Could you check a few things on this model? Use its own coordinates, in mm. Coordinates: 2 decimals unless noted, no trailing zeros. Order: outer loops, then holes, each group sorted by start corner. A loop starts at its lowest first (then second) coordinate and runs counter-clockwise, first axis right, second up. Notation, with made-up numbers: M -36.75,-28.5 L 6.25,-28.5 A19 ccw 6.25,-24.5 Z; hole C 26,-31 d8. An arc over 180 degrees is marked long. Put each result on its own line as item: value. Start each with the question number.
Solid Edge part; units mm, degrees
sketch "Sketch1" plane through (0, 0, 0) normal (0, 0, 1) x (1, 0, 0)
  line L0 (-0.1, 7.1216) -> (-0.1, 2.6716)
  line L1 (7.2, 2.6716) -> (-0.1, 2.6716)
  line L2 (7.2, 2.6716) -> (7.2, 0.455)
  line L3 (-0.1, 0.455) -> (7.2, 0.455)
  line L4 (-0.1, 0.455) -> (-0.1, 0)
  line L5 (9.2723, 0) -> (-0.1, 0)
  line L6 (6.623, 7.1216) -> (9.2723, 0)
  line L7 (6.623, 7.1216) -> (-0.1, 7.1216)
  dimension "D1" = 0.1
  dimension "D2" = 0.1
  dimension "D3" = 7.2
extrude "Protrusion1" add sketch "Sketch1" along normal blind 0.1
sketch "Sketch2" plane through (4.6037, 3.5608, 0.1) normal (0, 0, 1) x (1, 0, 0)
  line L0 (-2.7487, 0.3108) -> (-2.0887, 0.3108)
  line L1 (-2.0887, 0.3108) -> (-2.0887, 1.7108)
  line L2 (-2.0887, 1.7108) -> (-2.7487, 1.7108)
  line L3 (-2.7487, 1.7108) -> (-2.7487, 0.3108)
  line L4 (-1.9637, 0.3108) -> (-1.3037, 0.3108)
  line L5 (-1.3037, 0.3108) -> (-1.3037, 1.7108)
  line L6 (-1.3037, 1.7108) -> (-1.9637, 1.7108)
  line L7 (-1.9637, 1.7108) -> (-1.9637, 0.3108)
  line L8 (1.2163, 0.3108) -> (1.8763, 0.3108)
  line L9 (1.8763, 0.3108) -> (1.8763, 1.4908)
  line L10 (1.8763, 1.4908) -> (1.2163, 1.4908)
  line L11 (1.2163, 1.4908) -> (1.2163, 0.3108)
  line L12 (-3.5437, 0.3108) -> (-2.8837, 0.3108)
  line L13 (-2.8837, 0.3108) -> (-2.8837, 1.7108)
  line L14 (-2.8837, 1.7108) -> (-3.5437, 1.7108)
  line L15 (-3.5437, 1.7108) -> (-3.5437, 0.3108)
  dimension "D1" = 2.8837
  dimension "D2" = 3.5437
  dimension "D3" = 1.2163
extrude "Cutout1" cut sketch "Sketch2" against normal through all
Item 1: If we section it at D-D on y = 1.75: Write out the boundary of the cut face in (x, z).
Item 2: For pin 1 Ø1 at (x, y) = (2.5, 1) entering from +Z, with a flat end and sliding along its axis, tell me the tip position at first contact or that it passes through.
Item 3: If we section it at B-B on x = 3: Write out the boundary of the cut face in (y, z) (3 decimals), then the cut area to 4 significant figures.
Item 4: I need wall thicknesses on probe 1 along Y at (x, z) = (3.25, 0.05) (3 decimals); probe 2 along X at (y, z) = (1, 0.05); probe 3 along X at (y, z) = (6.25, 0.05). Which ranges of each line are inside material? Lowest first, please.
Item 5: If we section it at A-A on z = 0.05: Write out the boundary of the cut face in (x, y) (3 decimals).
Item 6: If we section it at C-C on x = 5.5: Write out the boundary of the cut face in (y, z) (3 decimals).
Geometry check:
1. outline: M 7.2,0 L 8.62,0 L 8.62,0.1 L 7.2,0.1 Z
2. pin 1: passes through
3. outline: M 0,0 L 0.455,0 L 0.455,0.1 L 0,0.1 Z; M 2.672,0 L 3.872,0 L 3.872,0.1 L 2.672,0.1 Z; M 5.272,0 L 7.122,0 L 7.122,0.1 L 5.272,0.1 Z
3. area: 0.3505 mm²
4. probe 1: y = 0 to 0.455, 2.672 to 3.872, 5.272 to 7.122
4. probe 2: x = 7.2 to 8.9
4. probe 3: x = -0.1 to 6.95
5. outline: M -0.1,0 L 9.272,0 L 6.623,7.122 L -0.1,7.122 L -0.1,2.672 L 7.2,2.672 L 7.2,0.455 L -0.1,0.455 Z; hole M 1.06,3.872 L 1.72,3.872 L 1.72,5.272 L 1.06,5.272 Z; hole M 1.855,3.872 L 2.515,3.872 L 2.515,5.272 L 1.855,5.272 Z; hole M 2.64,3.872 L 3.3,3.872 L 3.3,5.272 L 2.64,5.272 Z; hole M 5.82,3.872 L 6.48,3.872 L 6.48,5.052 L 5.82,5.052 Z
6. outline: M 0,0 L 0.455,0 L 0.455,0.1 L 0,0.1 Z; M 2.672,0 L 7.122,0 L 7.122,0.1 L 2.672,0.1 Z
